from build123d import *

# Parameters (mm, degrees)
SKETCH1_W           = 40
SKETCH1_H           = 20
BOSS_EXTRUDE1_DEPTH = 500
SKETCH3_W           = 38
SKETCH3_H           = 18
CUT_EXTRUDE1_DEPTH  = 501
CUT_EXTRUDE2_DEPTH  = 41


with BuildPart() as part:
    # Sketch1 → Boss-Extrude1 (new body)
    with BuildSketch(Plane.XY):
        with Locations((0, 2)):
            Rectangle(SKETCH1_W, SKETCH1_H)
    extrude(amount=BOSS_EXTRUDE1_DEPTH)

    # Sketch3 → Cut-Extrude1 (cut, through all)
    with BuildSketch(Plane.XY.offset(500)):
        with Locations((0, 2)):
            Rectangle(SKETCH3_W, SKETCH3_H)
    extrude(amount=-CUT_EXTRUDE1_DEPTH, mode=Mode.SUBTRACT)

    # Sketch4 → Cut-Extrude2 (cut, through all)
    with BuildSketch(Plane(origin=(20, 0, 0), x_dir=(0, 0, -1), z_dir=(1, 0, 0))):
        Polygon((-500, 12), (-480, 12), (-500, -8), align=None)
        Polygon((0, 12), (-20, 12), (0, -8), align=None)
    extrude(amount=-CUT_EXTRUDE2_DEPTH, mode=Mode.SUBTRACT)


solid = part.part
Model file for the job. Use its own axes, mm. A direction names the side the tool comes from. Give positions to 0.01 mm unless a question says otherwise; leave off trailing zeros. Loops run counter-clockwise (first coordinate to the right, second up) from the corner with the lowest first, then second, coordinate; pieces in that order, holes last. Notation, with made-up numbers: (-6, -31) - (19, -31) arc R23 ccw to (19, -17) - close; hole circle Ø6 at (-3.5, -35.5). An arc over 180 degrees is marked (long way). Use one line per item in the form item = value.
(1) Drill centre lines: L1, parallel to X at y = 9.5, z = 41.5; L2, parallel to Y at x = 16, z = 279. Where is each one in solid material? Low to high.
Determined:
L1 = -20 to -19, 19 to 20
L2 = -8 to -7, 11 to 12
(2) 3-axis set-ups, long thin cutter, end or side, ignore diameter. For faces 1 (the face through (-19, 2, 253)), 2 (the face through (0.1, 11.7, 480.3)): which of +Z, -Z, +X, -X, +Y, -Y reach the whole face in a straight line?
Determined:
face_1 = +Z, -Z
face_2 = +Z, +X, -X, +Y
(3) Pull direction Y, two halves, no side cores. Call faces 3 (the face through (0.1, 11.7, 19.7)), 4 (the face through (0, 11, 253)), 5 (the face through (20, 2, 246)): pulls with the +Y half, pulls with the -Y half, needs draft (parallel to the pull), parting line crosses it, or undercut.
Determined:
face_3 = pulls with the +Y half
face_4 = undercut
face_5 = needs draft
(4) Cut at B-B (x = 7). Give the cut face in (y, z).
Determined:
outline = (-8, 0) - (-7, 1) - (-7, 499) - (-8, 500) - close; (11, 19) - (12, 20) - (12, 480) - (11, 481) - close
(5) Cut at C-C (z = 271). Give the cut face in (x, y), then the cut area to 3 significant figures.
Determined:
outline = (-20, -8) - (20, -8) - (20, 12) - (-20, 12) - close; hole (-19, -7) - (19, -7) - (19, 11) - (-19, 11) - close
area = 116 mm^2
(6) Cut at A-A (y = -1). Give the cut face in (x, z).
Determined:
outline = (-20, 7) - (-19, 7) - (-19, 493) - (-20, 493) - close; (19, 7) - (20, 7) - (20, 493) - (19, 493) - close
